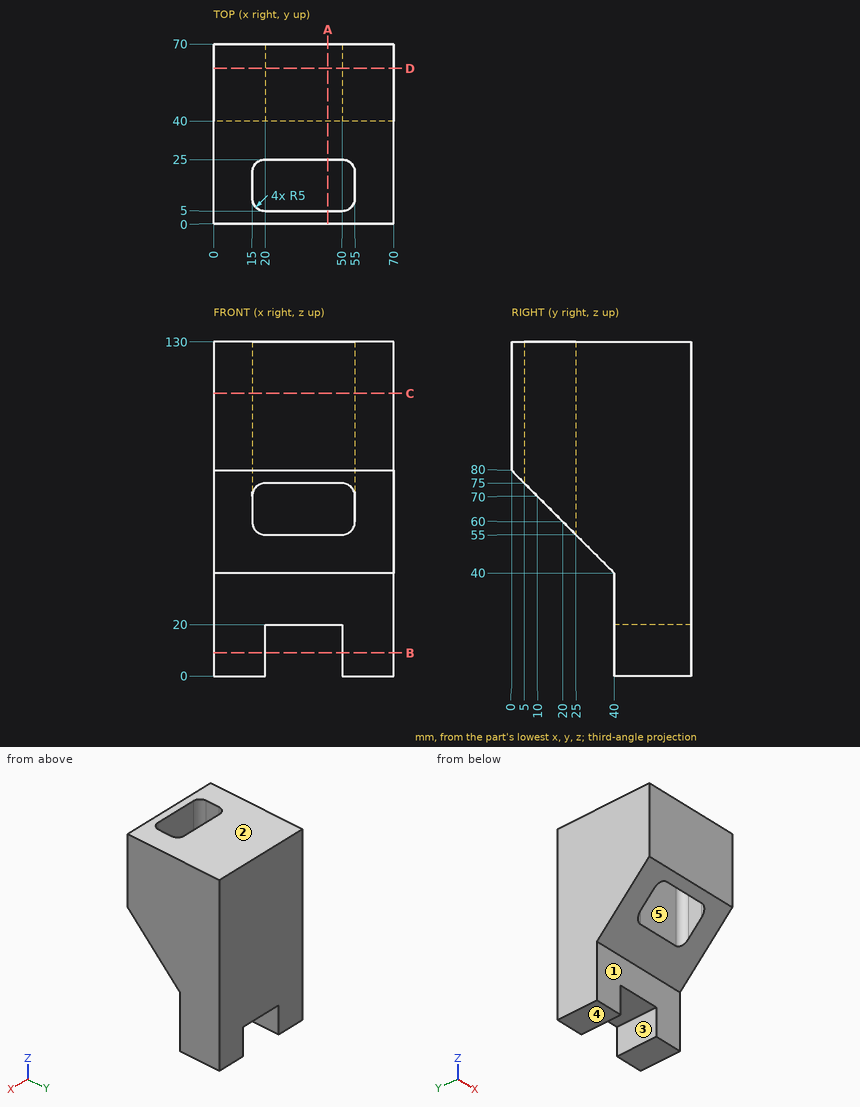
Print and shaded views of the part. All mm, measured from the part's lowest x, y and z. A direction names the side the tool comes from. Coordinates: 2 decimals unless noted, no trailing zeros. Loops run counter-clockwise (first coordinate to the right, second up) from the corner with the lowest first, then second, coordinate; pieces in that order, holes last. Notation, with made-up numbers: (53, 23.5) -> (86, 23.5) arc R11 cw to (86, 28.5) -> close; hole circle Ø6 at (4.5, -16.5). An arc over 180 degrees is marked (long way). Use a Markdown table: item, result. Add a question column.
Item 1: Flat gauge pins, fed straight in: P1, Ø5, axis at x = 20.5, y = 25.5, coming from the -Z side; P2, Ø2, axis at x = 61, y = 29, coming from the -Z side; P3, Ø12, axis at x = 50, z = 22, coming from the -Y side. Where does each tip first touch, or does it go through?
Item 2: Band-saw the part on C-C on z = 110. Write the cut outline in (x, y), plus the area to 3 significant figures.
Item 3: Band-saw the part on A-A on x = 44.5. Write the cut outline in (y, z), plus the area to 3 significant figures.
Item 4: Probe probe 1 along Y at (x, z) = (28.5, 120); probe 2 along X at (y, z) = (11.5, 69); probe 3 along Y at (x, z) = (66.5, 9). List the from-to ranges inside material, lowest first.
Item 5: Which spindle directions (+Z, -Z, +X, -X, +Y, -Y) get a long thin tool onto all of the face, cutting with end or side? Do the marked faces 1, 2, 3, 4 and 5. Say none if no direction does.
Item 6: Band-saw the part on B-B on z = 9. Write the cut outline in (x, y).
Item 7: Band-saw the part on D-D on y = 60.5. Write the cut outline in (x, z), plus the area to 3 significant figures.
Geometry says:
| question | item | result |
|---|---|---|
| 1 | P1 | z = 52 |
| 1 | P2 | z = 50 |
| 1 | P3 | y = 40 |
| 2 | outline | (0, 0) -> (70, 0) -> (70, 70) -> (0, 70) -> close; hole (15, 10) arc R5 ccw to (20, 5) -> (50, 5) arc R5 ccw to (55, 10) -> (55, 20) arc R5 ccw to (50, 25) -> (20, 25) arc R5 ccw to (15, 20) -> close |
| 2 | area | 4,120 mm² |
| 3 | outline | (0, 80) -> (5, 75) -> (5, 130) -> (0, 130) -> close; (25, 55) -> (40, 40) -> (40, 20) -> (70, 20) -> (70, 130) -> (25, 130) -> close |
| 3 | area | 4,800 mm² |
| 4 | probe 1 | 0 to 5, 25 to 70 |
| 4 | probe 2 | 0 to 15, 55 to 70 |
| 4 | probe 3 | 40 to 70 |
| 5 | face 1 | -Z, +X, -X, -Y |
| 5 | face 2 | +Z, +X, -X, +Y, -Y |
| 5 | face 3 | -Z, +Y, -Y |
| 5 | face 4 | -Z, +X, -X, +Y, -Y |
| 5 | face 5 | +Z, -Z |
| 6 | outline | (0, 40) -> (20, 40) -> (20, 70) -> (0, 70) -> close; (50, 40) -> (70, 40) -> (70, 70) -> (50, 70) -> close |
| 7 | outline | (0, 0) -> (20, 0) -> (20, 20) -> (50, 20) -> (50, 0) -> (70, 0) -> (70, 130) -> (0, 130) -> close |
| 7 | area | 8,500 mm² |
